```python
from build123d import *

# Parameters (mm, degrees)
SKETCH001_W        = 95
SKETCH001_H        = 95
PAD001_DEPTH       = 0.2
CHAMFER_SIZE       = 5
POCKET_DEPTH       = 5
POLARPATTERN_COUNT = 4
SKETCH007_W        = 129.60696
SKETCH007_H        = 24.349444
POCKET003_DEPTH    = 47.501


with BuildPart() as part:
    # Sketch001 → Pad001 (new body)
    with BuildSketch(Plane.XY):
        Rectangle(SKETCH001_W, SKETCH001_H)
    extrude(amount=-PAD001_DEPTH)

    # Chamfer
    chamfer_edges = [part.edges().sort_by_distance(p)[0] for p in [
        (-47.5, 47.5, -0.1),
        (47.5, 47.5, -0.1),
        (-47.5, -47.5, -0.1),
        (47.5, -47.5, -0.1),
    ]]
    chamfer(chamfer_edges, length=CHAMFER_SIZE)

    # Sketch003 (on Face2 of Chamfer) → Pocket (cut)
    with BuildSketch(Plane.XY):
        with BuildLine():
            ThreePointArc((-38, 44.5), (-39.5, 43), (-38, 41.5))
            Line((-38, 41.5), (38, 41.5))
            ThreePointArc((38, 41.5), (39.5, 43), (38, 44.5))
            Line((-38, 44.5), (38, 44.5))
        make_face()
    pocket = extrude(amount=-POCKET_DEPTH, mode=Mode.SUBTRACT)

    # PolarPattern: Pocket ×4 about axis
    polarpattern_axis = Axis((0, 0, 0), (0, 0, 1))
    for i in range(1, POLARPATTERN_COUNT):
        add(pocket.rotate(polarpattern_axis, i * 360 / POLARPATTERN_COUNT), mode=Mode.SUBTRACT)

    # Sketch007 → Pocket003 (cut, through all)
    with BuildSketch(Plane.YZ):
        with Locations((-2.349726, 5.652762)):
            Rectangle(SKETCH007_W, SKETCH007_H)
    extrude(amount=-POCKET003_DEPTH, mode=Mode.SUBTRACT)


solid = part.part
```
Geometry check sheet. Reference: the model listing, model coordinates, mm. Round coordinates to 2 decimals unless told otherwise and drop trailing zeros. Loops run counter-clockwise (first coordinate to the right, second up) from the corner with the lowest first, then second, coordinate; pieces in that order, holes last. Notation, with made-up numbers: (86, 71) - (125, 71) arc R23 ccw to (125, 90) - close; hole circle Ø10 at (57, -13.75). An arc over 180 degrees is marked (long way). Use a Markdown table: item, result.
Q1. Go/stop test with a flat-tipped pin: P1, Ø6, axis at x = 20.5, y = 7, coming from the +Z side. Record where the tip stops, or that it passes through.
Solutions:
| item | result |
|---|---|
| P1 | stops at z = 0 |
Q2. Cross-section at C-C on z = -0.1. Record the cut outline in (x, y), plus the area to 3 significant figures.
Solutions:
| item | result |
|---|---|
| outline | (0, -47.5) - (42.5, -47.5) - (47.5, -42.5) - (47.5, 42.5) - (42.5, 47.5) - (0, 47.5) - (0, 44.5) - (38, 44.5) arc R1.5 cw to (38, 41.5) - (0, 41.5) - (0, -41.5) - (38, -41.5) arc R1.5 cw to (38, -44.5) - (0, -44.5) - close; hole (41.5, -38) arc R1.5 ccw to (44.5, -38) - (44.5, 38) arc R1.5 ccw to (41.5, 38) - close |
| area | 4,020 mm2 |
Q3. Material ranges on line 1 (Y direction, x = 21, z = -0.05); line 2 (X direction, y = -21.5, z = -0.05); line 3 (Y direction, x = 42, z = -0.05), recorded low to high.
Solutions:
| item | result |
|---|---|
| line 1 | y = -47.5 to -44.5, -41.5 to 41.5, 44.5 to 47.5 |
| line 2 | x = 0 to 41.5, 44.5 to 47.5 |
| line 3 | y = -47.5 to -39.12, 39.12 to 47.5 |
Q4. Cross-section at A-A on x = 12.5. Record the cut outline in (y, z), plus the area to 3 significant figures.
Solutions:
| item | result |
|---|---|
| outline | (-47.5, -0.2) - (-44.5, -0.2) - (-44.5, 0) - (-47.5, 0) - close; (-41.5, -0.2) - (41.5, -0.2) - (41.5, 0) - (-41.5, 0) - close; (44.5, -0.2) - (47.5, -0.2) - (47.5, 0) - (44.5, 0) - close |
| area | 17.8 mm2 |
Q5. Cross-section at B-B on y = 25.5. Record the cut outline in (x, z).
Solutions:
| item | result |
|---|---|
| outline | (0, -0.2) - (41.5, -0.2) - (41.5, 0) - (0, 0) - close; (44.5, -0.2) - (47.5, -0.2) - (47.5, 0) - (44.5, 0) - close |
